Solid Edge part; units mm, degrees
sketch "Sketch1" plane through (0, 0, 0) normal (0, 0, 1) x (1, 0, 0)
  line L0 (0, 3.1177) -> (2.7, 1.5588)
  line L1 (2.7, 1.5588) -> (2.7, -1.5588)
  line L2 (2.7, -1.5588) -> (0, -3.1177)
  line L3 (0, -3.1177) -> (-2.7, -1.5588)
  line L4 (-2.7, -1.5588) -> (-2.7, 1.5588)
  line L5 (-2.7, 1.5588) -> (0, 3.1177)
extrude "Protrusion1" add sketch "Sketch1" along normal blind 2.4
hole "Hole_1" at (0, 0, 2.4) direction (0, 0, -1) diameter 3 end up to next
Read the model definition and answer for the solid it produces. Units are mm, in the model's axes. Give positions to 0.01 mm unless a question says otherwise; leave off trailing zeros. Loops run counter-clockwise (first coordinate to the right, second up) from the corner with the lowest first, then second, coordinate; pieces in that order, holes last. Notation, with made-up numbers: (39.25, 12) - (67.25, 12) arc R28 ccw to (67.25, 35) - close; hole circle Ø7 at (76.5, 15.25). An arc over 180 degrees is marked (long way). Answer as CSV lines item,"result". Start each with the question number.
1) Find section C-C (x = -0.9). Write down the section's boundary in (y, z), then the cut area to 3 significant figures.
2) This flat-tipped pin is pushed along its axis until it touches: pin 1 Ø3 at (x, y) = (-0.5, 1.5) entering from -Z. Where does it stop, or does it pass through?
3) Find section A-A (y = 0). Write down the section's boundary in (x, z).
4) Find section D-D (y = 2.75). Write down the section's boundary in (x, z).
5) Determine the mould class of faces 1 (the face through (-1.2, -1.3, 2.4)), 2 (the face through (0.07, 1.5, 1.22)), 3 (the face through (-1.33, -2.35, 1.18)) for opening direction X: released by +X, released by -X, zero draft, split by the parting line, or undercut.
6) Straight lines are drawn through the part: L1, parallel to X at y = 0, z = 1.65; L2, parallel to Y at x = 1.1, z = 2; L3, parallel to Y at x = 0.3, z = 0.5. For each, find the intervals that lie inside material, in ascending order. Write a range as from..to.
7) Find section B-B (z = 0.3). Write down the section's boundary in (x, y).
Findings below:
1,outline,"(-2.6, 0) - (-1.2, 0) - (-1.2, 2.4) - (-2.6, 2.4) - close; (1.2, 0) - (2.6, 0) - (2.6, 2.4) - (1.2, 2.4) - close"
1,area,"6.71 mm^2"
2,pin 1,"z = 0"
3,outline,"(-2.7, 0) - (-1.5, 0) - (-1.5, 2.4) - (-2.7, 2.4) - close; (1.5, 0) - (2.7, 0) - (2.7, 2.4) - (1.5, 2.4) - close"
4,outline,"(-0.64, 0) - (0.64, 0) - (0.64, 2.4) - (-0.64, 2.4) - close"
5,face 1,"zero draft"
5,face 2,"undercut"
5,face 3,"released by -X"
6,L1,"-2.7..-1.5, 1.5..2.7"
6,L2,"-2.48..-1.02, 1.02..2.48"
6,L3,"-2.94..-1.47, 1.47..2.94"
7,outline,"(-2.7, -1.56) - (0, -3.12) - (2.7, -1.56) - (2.7, 1.56) - (0, 3.12) - (-2.7, 1.56) - close; hole circle Ø3 at (0, 0)"
